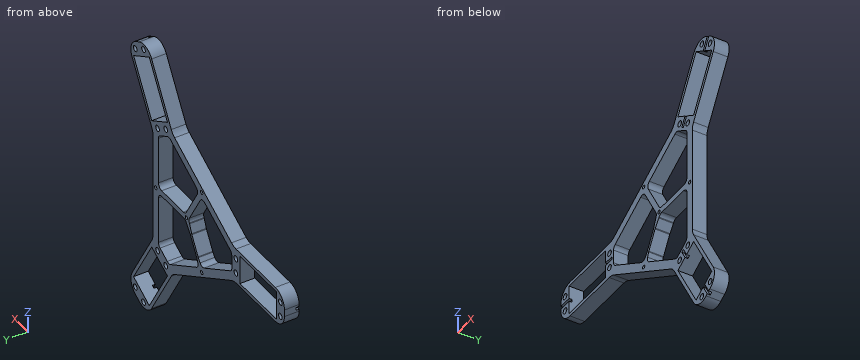
from build123d import *

# Parameters (mm, degrees)
SKETCH1_R           = 2
SKETCH1_R_2         = 1.25
SKETCH1_W           = 40
SKETCH1_H           = 20
BOSS_EXTRUDE1_DEPTH = 10
SKETCH2_W           = 2
SKETCH2_H           = 4
CUT_EXTRUDE1_DEPTH  = 56
SKETCH3_W           = 2
SKETCH3_H           = 4
CUT_EXTRUDE2_DEPTH  = 56
SKETCH4_W           = 2
SKETCH4_H           = 4
CUT_EXTRUDE3_DEPTH  = 56
FILLET1_R           = 10
FILLET2_R           = 3.5


with BuildPart() as part:
    # Sketch1 → Boss-Extrude1 (new body)
    with BuildSketch(Plane(origin=(0, 0, 0), x_dir=(1, 0, 0), z_dir=(0, 1, 0))):
        Polygon((-9, 22.4), (-9, -2.4), (47, -2.4), (114.261284993, -41.233320997), (142.261284993, -89.730743609), (163.738715007, -77.330743609), (135.738715007, -28.833320997), (135.738715007, 48.833320997), (163.738715007, 97.330743609), (142.261284993, 109.730743609), (114.261284993, 61.233320997), (47, 22.4), align=None)
        with Locations(Location((-4.5, 4.8, 0), (0, 0, 270))):
            Circle(SKETCH1_R, mode=Mode.SUBTRACT)
        with Locations(Location((44.5, 4.8, 0), (0, 0, 270))):
            Circle(SKETCH1_R, mode=Mode.SUBTRACT)
        with Locations(Location((146.2466679, -82.233629292, 0), (0, 0, 270))):
            Circle(SKETCH1_R, mode=Mode.SUBTRACT)
        with Locations(Location((155.2533321, -77.033629292, 0), (0, 0, 270))):
            Circle(SKETCH1_R, mode=Mode.SUBTRACT)
        with Locations(Location((121.7466679, -39.798384506, 0), (0, 0, 270))):
            Circle(SKETCH1_R, mode=Mode.SUBTRACT)
        Polygon((157.160254038, -70.736514975), (139.839745962, -80.736514975), (119.839745962, -46.095498823), (137.160254038, -36.095498823), align=None, mode=Mode.SUBTRACT)
        with Locations(Location((82.130642497, -19.218584287, 0), (0, 0, 270))):
            Circle(SKETCH1_R_2, mode=Mode.SUBTRACT)
        Polygon((85.362693304, -17.620508076), (100.154700538, 8), (129.738715007, 8), (129.738715007, -29.988021535), (118.261284993, -36.614518843), align=None, mode=Mode.SUBTRACT)
        with Locations(Location((130.7533321, -34.598384506, 0), (0, 0, 270))):
            Circle(SKETCH1_R, mode=Mode.SUBTRACT)
        with Locations(Location((-4.5, 15.2, 0), (0, 0, 270))):
            Circle(SKETCH1_R, mode=Mode.SUBTRACT)
        with Locations((20, 10)):
            Rectangle(SKETCH1_W, SKETCH1_H, mode=Mode.SUBTRACT)
        with Locations(Location((44.5, 15.2, 0), (0, 0, 270))):
            Circle(SKETCH1_R, mode=Mode.SUBTRACT)
        Polygon((95.535898385, 12), (96.690598923, 10), (81.898591689, -15.620508076), (49, 3.373502692), (49, 16.626497308), (82.014634361, 35.687505343), (85.99611255, 30.523393759), (93.064765898, 18.280127019), align=None, mode=Mode.SUBTRACT)
        with Locations(Location((99, 10, 0), (0, 0, 270))):
            Circle(SKETCH1_R_2, mode=Mode.SUBTRACT)
        with Locations(Location((82.130642497, 39.218584287, 0), (0, 0, 270))):
            Circle(SKETCH1_R_2, mode=Mode.SUBTRACT)
        Polygon((129.738715007, 49.988021535), (129.738715007, 12), (100.154700538, 12), (99, 14), (94.796816706, 19.280127019), (87.728163358, 31.523393759), (85.246650633, 37.553510808), (118.261284993, 56.614518843), align=None, mode=Mode.SUBTRACT)
        with Locations(Location((132.738715007, 10, 0), (0, 0, 270))):
            Circle(SKETCH1_R_2, mode=Mode.SUBTRACT)
        with Locations(Location((130.7533321, 54.598384506, 0), (0, 0, 270))):
            Circle(SKETCH1_R, mode=Mode.SUBTRACT)
        with Locations(Location((121.7466679, 59.798384506, 0), (0, 0, 270))):
            Circle(SKETCH1_R, mode=Mode.SUBTRACT)
        Polygon((119.839745962, 66.095498823), (139.839745962, 100.736514975), (157.160254038, 90.736514975), (137.160254038, 56.095498823), align=None, mode=Mode.SUBTRACT)
        with Locations(Location((146.2466679, 102.233629292, 0), (0, 0, 270))):
            Circle(SKETCH1_R, mode=Mode.SUBTRACT)
        with Locations(Location((155.2533321, 97.033629292, 0), (0, 0, 270))):
            Circle(SKETCH1_R, mode=Mode.SUBTRACT)
    extrude(amount=BOSS_EXTRUDE1_DEPTH)

    # Sketch2 → Cut-Extrude1 (cut)
    with BuildSketch(Plane.ZY.offset(9)):
        with Locations((-10, 0)):
            Rectangle(SKETCH2_W, SKETCH2_H)
    extrude(amount=-CUT_EXTRUDE1_DEPTH, mode=Mode.SUBTRACT)

    # Sketch3 → Cut-Extrude2 (cut)
    with BuildSketch(Plane(origin=(74.419872981, 0, 128.899001096), x_dir=(0.8660254037844434, 0, -0.49999999999999173), z_dir=(0.49999999999999173, 0, 0.8660254037844434))):
        with Locations((90.736514975, 0)):
            Rectangle(SKETCH3_W, SKETCH3_H)
    extrude(amount=-CUT_EXTRUDE2_DEPTH, mode=Mode.SUBTRACT)

    # Sketch4 → Cut-Extrude3 (cut)
    with BuildSketch(Plane(origin=(83.080127019, 0, -143.899001096), x_dir=(-0.8660254037844363, 0, -0.5000000000000043), z_dir=(0.5000000000000043, 0, -0.8660254037844363))):
        with Locations((-80.736514975, 0)):
            Rectangle(SKETCH4_W, SKETCH4_H)
    extrude(amount=-CUT_EXTRUDE3_DEPTH, mode=Mode.SUBTRACT)

    # Fillet1
    fillet1_edges = [part.edges().sort_by_distance(p)[0] for p in [
        (135.738715007, 5, 28.833320997),
        (163.738715007, 5, 77.330743609),
        (142.261284993, 5, 89.730743609),
        (114.261284993, 5, 41.233320997),
        (47, 5, 2.4),
        (-9, 5, 2.4),
        (-9, 5, -22.4),
        (47, 5, -22.4),
        (114.261284993, 5, -61.233320997),
        (142.261284993, 5, -109.730743609),
        (163.738715007, 5, -97.330743609),
        (135.738715007, 5, -48.833320997),
    ]]
    fillet(fillet1_edges, radius=FILLET1_R)

    # Fillet2
    fillet2_edges = [part.edges().sort_by_distance(p)[0] for p in [
        (49, 5, -16.626497308),
        (49, 5, -3.373502692),
        (81.898591689, 5, 15.620508076),
        (96.690598923, 5, -10),
        (95.535898385, 5, -12),
        (93.064765898, 5, -18.280127019),
        (85.99611255, 5, -30.523393759),
        (82.014634361, 5, -35.687505343),
        (87.728163358, 5, -31.523393759),
        (94.796816706, 5, -19.280127019),
        (99, 5, -14),
        (100.154700538, 5, -12),
        (129.738715007, 5, -12),
        (129.738715007, 5, -49.988021535),
        (118.261284993, 5, -56.614518843),
        (85.246650633, 5, -37.553510808),
        (100.154700538, 5, -8),
        (85.362693304, 5, 17.620508076),
        (118.261284993, 5, 36.614518843),
        (129.738715007, 5, 29.988021535),
        (129.738715007, 5, -8),
    ]]
    fillet(fillet2_edges, radius=FILLET2_R)


solid = part.part
Source: CAD feature listing. Evaluate the final solid. Frame: model axes, mm. Coordinates: 2 decimals unless noted, no trailing zeros. Loops run counter-clockwise (first coordinate to the right, second up) from the corner with the lowest first, then second, coordinate; pieces in that order, holes last. Notation, with made-up numbers: (-10.75, -38.5) - (18.25, -38.5) arc R28 cw to (18.25, -20.5) - close; hole circle Ø7 at (87, 48.25). An arc over 180 degrees is marked (long way). Return JSON: item names as keys, results as strings.
Q1. Section A-A, the plane x = 23. Return loops of the section in (y, z).
Results:
{"outline": "(0, -22.4) - (10, -22.4) - (10, -20) - (0, -20) - close; (0, 0) - (10, 0) - (10, 2.4) - (0, 2.4) - close"}
Q2. Contact query for flat-ended pins moving along their axis: P1, Ø2, axis at x = 42, y = 1.5, coming from the -Z side; P2, Ø3.5, axis at x = -4.5, z = -4.8, coming from the -Y side; P3, Ø5, axis at x = 155.25, z = -97.03, coming from the +Y side; P4, Ø2, axis at y = 6.5, z = -71, coming from the +X side. Output: stop coordinate, or through.
Results:
{"P1": "z = -22.4", "P2": "through", "P3": "y = 10", "P4": "x = 149.11"}
Q3. Material intervals for line 1 along X through (y, z) = (7, -10); line 2 along X through (y, z) = (7, -26); line 3 along X through (y, z) = (8.25, -25.5), sorted ascending.
Results:
{"line 1": "-9 to 0, 40 to 49, 96.15 to 97.75, 100.25 to 131.49, 133.99 to 135.74", "line 2": "53.24 to 65.24, 88.61 to 90.92, 129.74 to 135.74", "line 3": "52.37 to 64.37, 88.9 to 91.21, 129.74 to 135.74"}
Q4. Section C-C, the plane y = 7. Give the number of separate pieces and of enclosed holes in the cut face, plus the area to 3 significant figures.
Results:
{"separate pieces": "1", "enclosed holes": "22", "area": "3,340 mm2"}
Q5. Section B-B, the plane z = -84.5. Return loops of the section in (x, y), plus the area to 3 significant figures.
Results:
{"outline": "(127.69, 0) - (130.47, 0) - (130.47, 10) - (127.69, 10) - close; (153.56, 0) - (156.33, 0) - (156.33, 10) - (153.56, 10) - close", "area": "55.4 mm2"}
